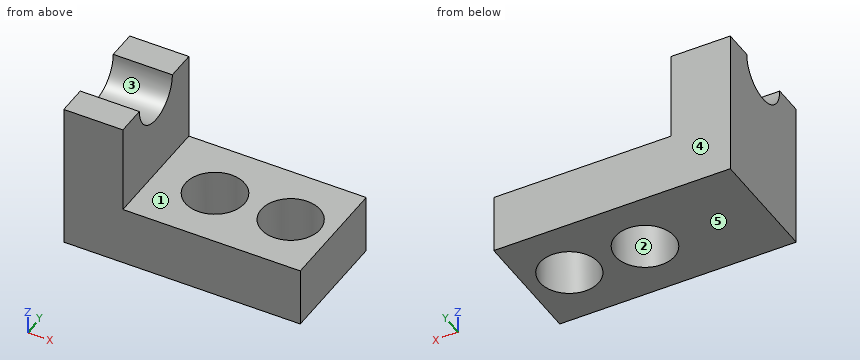
```python
from build123d import *

# Parameters (mm, degrees)
F1_DEPTH = 50.8
F3_DEPTH = 80.264
F4_R     = 12.7
F4_R_2   = 12.625616
F5_DEPTH = 50.8


with BuildPart() as f1:
    # F0 (on Front) → F1 (new body)
    with BuildSketch(Plane.XZ):
        Polygon((-18.470924, 25.060495), (-43.870924, 25.060495), (-43.870924, -38.439505), (57.729076, -38.439505), (57.729076, -13.039505), (-18.470924, -13.039505), align=None)
    extrude(amount=F1_DEPTH)

    # F2 (on face) → F3 (cut)
    with BuildSketch(Plane.YZ.offset(-18.470924)):
        with BuildLine():
            Line((-12.7, 25.060495), (-38.1, 25.060495))
            ThreePointArc((-38.1, 25.060495), (-25.4, 12.360495), (-12.7, 25.060495))
        make_face()
    extrude(amount=-F3_DEPTH, mode=Mode.SUBTRACT)

    # F4 (on face) → F5 (cut)
    with BuildSketch(Plane.XY.offset(-13.039505)):
        with Locations((6.929076, -25.4)):
            Circle(F4_R)
        with Locations((39.437555, -25.4)):
            Circle(F4_R_2)
    extrude(amount=-F5_DEPTH, mode=Mode.SUBTRACT)


solid = f1.part
```
Read the model definition and answer for the solid it produces. Units are mm, in the model's axes. Face numbers are marked on the shaded views. A direction names the side the tool comes from. Round coordinates to 2 decimals unless told otherwise and drop trailing zeros. Write each loop counter-clockwise with the first axis right and the second up, starting at its lowest first coordinate (ties: lowest second). Pieces come first, ordered by that corner, then holes. Notation, with made-up numbers: (53, 73) -> (84, 73) arc R16 cw to (84, 83) -> close; hole circle Ø4 at (19, -4). An arc over 180 degrees is marked (long way). Answer in a Markdown table with one row per item. Add a question column.
1) Given P1, Ø2, axis at x = 37.5, y = -44.5, coming from the +Z side; P2, Ø19, axis at y = -33.5, z = 15, coming from the +X side, each flat-ended and moving along its own axis, determine where each tip first touches the part or whether it passes through.
2) Determine the mould class of the marked faces 3, 4 and 5 for opening direction Y: pulls with the +Y half, pulls with the -Y half, needs draft (parallel to the pull), parting line crosses it, or undercut.
3) Consider line 1 (X direction, y = -25, z = -25); line 2 (X direction, y = -36, z = -34); line 3 (Z direction, x = -14, y = -31.5). Determine where each line is inside the solid, lowest interval first.
4) Find section B-B, the plane z = -27. Determine the outline of the cut face in (x, y).
5) Which of the six approach directions +Z, -Z, +X, -X, +Y, -Y give full straight-line access (tool end or side, diameter ignored) to the marked faces 1 and 2?
6) Find section D-D, the plane z = 16. Determine the outline of the cut face in (x, y), and give its area (3 significant figures).
7) Find section A-A, the plane y = -25.4. Determine the outline of the cut face in (x, z), and give its area (3 significant figures).
8) Find section C-C, the plane y = -43.5. Determine the outline of the cut face in (x, z), and give its area (3 significant figures).
Findings below:
| question | item | result |
|---|---|---|
| 1 | P1 | z = -13.04 |
| 1 | P2 | x = -18.47 |
| 2 | face 3 | undercut |
| 2 | face 4 | pulls with the +Y half |
| 2 | face 5 | needs draft |
| 3 | line 1 | -43.87 to -5.76, 19.62 to 26.82, 52.06 to 57.73 |
| 3 | line 2 | -43.87 to -0.07, 13.92 to 32.58, 46.3 to 57.73 |
| 3 | line 3 | -38.44 to -13.04 |
| 4 | outline | (-43.87, -50.8) -> (57.73, -50.8) -> (57.73, 0) -> (-43.87, 0) -> close; hole circle Ø25.4 at (6.93, -25.4); hole circle Ø25.25 at (39.44, -25.4) |
| 5 | face 1 | +Z, +X, +Y, -Y |
| 5 | face 2 | +Z, -Z |
| 6 | outline | (-43.87, -50.8) -> (-18.47, -50.8) -> (-18.47, -34.3) -> (-43.87, -34.3) -> close; (-43.87, -16.5) -> (-18.47, -16.5) -> (-18.47, 0) -> (-43.87, 0) -> close |
| 6 | area | 838 mm² |
| 7 | outline | (-43.87, -38.44) -> (-5.77, -38.44) -> (-5.77, -13.04) -> (-18.47, -13.04) -> (-18.47, 12.36) -> (-43.87, 12.36) -> close; (19.63, -38.44) -> (26.81, -38.44) -> (26.81, -13.04) -> (19.63, -13.04) -> close; (52.06, -38.44) -> (57.73, -38.44) -> (57.73, -13.04) -> (52.06, -13.04) -> close |
| 7 | area | 1,940 mm² |
| 8 | outline | (-43.87, -38.44) -> (57.73, -38.44) -> (57.73, -13.04) -> (-18.47, -13.04) -> (-18.47, 25.06) -> (-43.87, 25.06) -> close |
| 8 | area | 3,550 mm² |
